Could you check a few things on this model? Use its own coordinates, in mm. A direction names the side the tool comes from. Give positions to 0.01 mm unless a question says otherwise; leave off trailing zeros. Loops run counter-clockwise (first coordinate to the right, second up) from the corner with the lowest first, then second, coordinate; pieces in that order, holes last. Notation, with made-up numbers: M 50.5,-7 L 95.5,-7 A14 ccw 95.5,16 Z; hole C 77.25,60.25 d6. An arc over 180 degrees is marked long. Use CSV: the item, a comma, the result in double quotes.
```python
from build123d import *

# Parameters (mm, degrees)
PAD_DEPTH     = 3.81
SKETCH001_R   = 1.7
HOLE_DEPTH    = 24.892
SKETCH002_R   = 0.8
HOLE001_DEPTH = 24.892


with BuildPart() as part:
    # Sketch → Pad (new body)
    with BuildSketch(Plane.XY):
        Polygon((-43.053, 0), (-43.053, -7.62), (-36.068, -7.62), (-36.068, -3.81), (36.068, -3.81), (36.068, -7.62), (43.053, -7.62), (43.053, 0), align=None)
    extrude(amount=PAD_DEPTH)

    # Sketch001 (on Face10 of Pad) → Hole (cut)
    with BuildSketch(Plane.XY.offset(3.81)):
        with Locations((-39.5605, -4.826)):
            Circle(SKETCH001_R)
        with Locations((39.5605, -4.826)):
            Circle(SKETCH001_R)
    extrude(amount=-HOLE_DEPTH, mode=Mode.SUBTRACT)

    # Sketch002 (on Face5 of Hole) → Hole001 (cut)
    with BuildSketch(Plane.XY.offset(3.81)):
        with Locations((-8.89, -1.905)):
            Circle(SKETCH002_R)
        with Locations((8.89, -1.905)):
            Circle(SKETCH002_R)
    extrude(amount=-HOLE001_DEPTH, mode=Mode.SUBTRACT)


solid = part.part
```
1. Please list where these lines run through material, in increasing order: line 1 (X direction, y = -5, z = 2.1); line 2 (Y direction, x = -8.89, z = 1.4) (3 decimals); line 3 (X direction, y = -5.5, z = 0.55).
Outcome:
line 1,"-43.05 to -41.25, -37.87 to -36.07, 36.07 to 37.87, 41.25 to 43.05"
line 2,"-3.81 to -2.705, -1.105 to 0"
line 3,"-43.05 to -41.12, -38 to -36.07, 36.07 to 38, 41.12 to 43.05"
2. I want a section at D-D, the plane x = -7. List the corners of the cut face in (y, z) for me, then the cut area to 3 significant figures.
Outcome:
outline,"M -3.81,0 L 0,0 L 0,3.81 L -3.81,3.81 Z"
area,"14.5 mm2"
3. I want a section at A-A, the plane x = 8.89. List the corners of the cut face in (y, z) for me (3 decimals), then the cut area to 3 significant figures.
Outcome:
outline,"M -3.81,0 L -2.705,0 L -2.705,3.81 L -3.81,3.81 Z; M -1.105,0 L 0,0 L 0,3.81 L -1.105,3.81 Z"
area,"8.42 mm2"
4. I'm going to push flat-ended pins straight in: pin 1 Ø1 at (x, z) = (9, 2) entering from +Y; pin 2 Ø1.1 at (x, z) = (0.5, 1) entering from -Y. Where does each tip first touch, or does it pass through?
Outcome:
pin 1,"y = 0"
pin 2,"y = -3.81"
5. Which directions (+Z, -Z, +X, -X, +Y, -Y) give clear straight access to the entire face, cutting with the end or side of a thin tool? Please do faces 1 (the face through (41.182, -4.315, 1.932)), 2 (the face through (36.068, -6, 2)).
Outcome:
face 1,"+Z, -Z"
face 2,"+Z, -Z, -Y"
6. If we mould it in two halves opening along X, with no side actions, what happens to faces 3 (the face through (-40.813, -3.677, 1.932)), 4 (the face through (8.3, -1.364, 1.932)), 5 (the face through (1, 0, 2)), 6 (the face through (-43.053, -4, 2))? For each: +X half, -X half, draft (parallel to the pull), parting line (faces both ways), or undercut.
Outcome:
face 3,"undercut"
face 4,"undercut"
face 5,"draft"
face 6,"-X half"
7. I want a section at C-C, the plane z = 1.3. List the corners of the cut face in (x, y) for me (1 decimal).
Outcome:
outline,"M -43.1,-7.6 L -36.1,-7.6 L -36.1,-3.8 L 36.1,-3.8 L 36.1,-7.6 L 43.1,-7.6 L 43.1,0 L -43.1,0 Z; hole C -39.6,-4.8 d3.4; hole C -8.9,-1.9 d1.6; hole C 8.9,-1.9 d1.6; hole C 39.6,-4.8 d3.4"
8. I want a section at B-B, the plane y = -5.75. List the corners of the cut face in (x, z) for me, then the cut area to 3 significant figures.
Outcome:
outline,"M -43.05,0 L -40.99,0 L -40.99,3.81 L -43.05,3.81 Z; M -38.13,0 L -36.07,0 L -36.07,3.81 L -38.13,3.81 Z; M 36.07,0 L 38.13,0 L 38.13,3.81 L 36.07,3.81 Z; M 40.99,0 L 43.05,0 L 43.05,3.81 L 40.99,3.81 Z"
area,"31.5 mm2"
